Can you work these out from the model? Positions are in its coordinate system, mm. Coordinates: 2 decimals unless noted, no trailing zeros. Write each loop counter-clockwise with the first axis right and the second up, starting at its lowest first coordinate (ties: lowest second). Pieces come first, ordered by that corner, then holes. Notation, with made-up numbers: (58.25, -31) -> (105.25, -31) arc R31 ccw to (105.25, 0) -> close; hole circle Ø5 at (21, 48). An arc over 180 degrees is marked (long way). Use one line per item in the form item = value.
```python
from build123d import *


with BuildPart() as f1:
    # F0 (on Front) → F1 (revolve)
    with BuildSketch(Plane.XZ):
        Polygon((7.89093, 157.690874), (-42.10907, 157.690874), (-52.10907, 148.301338), (-42.10907, 137.651184), (-52.10907, 128.261649), (-42.10907, 117.611494), (-52.10907, 108.221959), (-42.10907, 97.571805), (-52.10907, 88.182269), (-42.10907, 77.532115), (-52.10907, 68.14258), (-42.10907, 57.492426), (-52.10907, 48.10289), (-42.10907, 37.452736), (-52.10907, 28.063201), (-42.10907, 17.413046), (-52.10907, 8.023511), (-42.10907, -2.626643), (-52.10907, -12.016179), (-42.10907, -22.666333), (-52.10907, -32.055868), (-42.10907, -42.706022), (-52.10907, -52.095558), (-42.10907, -62.745712), (-52.10907, -72.135247), (-42.10907, -82.785402), (-52.10907, -92.174937), (-42.10907, -102.825091), (-52.10907, -112.214627), (-42.10907, -122.864781), (-52.10907, -132.254316), (-42.10907, -142.90447), (-52.10907, -152.294006), (-42.10907, -162.94416), (-52.10907, -172.333695), (-42.10907, -182.983849), (-52.10907, -191.579593), (7.89093, -191.579593), align=None)
    revolve(axis=Axis((7.89093, 0, -16.94436), (0, 0, -1)))


solid = f1.part
```
Q1. Will these pins go through, and if not, where does the flat tip stop? pin 1 (8 mm diameter, centred on x = 30, z = -144.5, fed in from -Y); pin 2 (2 mm diameter, centred on y = 1.5, z = 89, fed in from -X); pin 3 (4 mm diameter, centred on y = -16, z = -77, fed in from +X).
Return value:
pin_1 = -51.7
pin_2 = -52.1
pin_3 = 63
Q2. Thinking about a two-plate mould opening in Z: for faces 1 (the conical face through (-15.47, -44.91, 56.91)), 2 (the flat face through (7, 1, 157.691)), 3 (the flat face through (9, 1, -191.58)), which applies, released by +Z, released by -Z, zero draft, split by the parting line, or undercut?
Return value:
face_1 = undercut
face_2 = released by +Z
face_3 = released by -Z
Q3. Suppose I cut it at B-B (z = -136). Write out the boundary of the cut face in (x, y), then the cut area to 3 significant figures.
Return value:
outline = circle Ø112.97 at (7.89, 0)
area = 10,000 mm2
Q4. If I drill on line 1 (Y direction, x = -34, z = 90); line 2 (Y direction, x = -41.5, z = -10.5); line 3 (X direction, y = -3.5, z = 3), over which ranges is the centre line in solid material (lowest first)? Write a range as from..to.
Return value:
line_1 = -40.21..40.21
line_2 = -31.13..31.13
line_3 = -47.28..63.06
Q5. Suppose I cut it at A-A (z = 133). Write out the boundary of the cut face in (x, y), then the cut area to 3 significant figures.
Return value:
outline = circle Ø109.91 at (7.89, 0)
area = 9,490 mm2
